from build123d import *

# Parameters (mm, degrees)
SKETCH_1_W          = 15
SKETCH_1_H          = 15
SKETCH_1_W_2        = 13
SKETCH_1_H_2        = 13
EXTRUDE_1_DEPTH     = 390
SKETCH_2_R          = 1.45
CUT_EXTRUDE_1_DEPTH = 391.36041039
SKETCH_3_R          = 1.45
CUT_EXTRUDE_2_DEPTH = 391.36041039


with BuildPart() as part:
    # 草图1 → 凸台-拉伸1 (new body)
    with BuildSketch(Plane(origin=(0, 0, 0), x_dir=(0, 0, -1), z_dir=(1, 0, 0))):
        Rectangle(SKETCH_1_W, SKETCH_1_H)
        Rectangle(SKETCH_1_W_2, SKETCH_1_H_2, mode=Mode.SUBTRACT)
    extrude(amount=EXTRUDE_1_DEPTH)

    # 草图2 → 切除-拉伸1 (cut, through all)
    with BuildSketch(Plane(origin=(0, 0, -7.5), x_dir=(-1, 0, 0), z_dir=(0, 0, -1))):
        with Locations((-366, 0)):
            Circle(SKETCH_2_R)
        with Locations((-376, 0)):
            Circle(SKETCH_2_R)
        with Locations((-19, 0)):
            Circle(SKETCH_2_R)
        with Locations((-9, 0)):
            Circle(SKETCH_2_R)
    extrude(amount=-CUT_EXTRUDE_1_DEPTH, mode=Mode.SUBTRACT)

    # 草图3 → 切除-拉伸2 (cut, through all)
    with BuildSketch(Plane(origin=(0, 7.5, 0), x_dir=(1, 0, 0), z_dir=(0, 1, 0))):
        with Locations(Location((371, 0, 0), (0, 0, 270))):
            Circle(SKETCH_3_R)
        with Locations(Location((381, 0, 0), (0, 0, 270))):
            Circle(SKETCH_3_R)
        with Locations(Location((14, 0, 0), (0, 0, 270))):
            Circle(SKETCH_3_R)
        with Locations(Location((177, 0, 0), (0, 0, 270))):
            Circle(SKETCH_3_R)
        with Locations(Location((187, 0, 0), (0, 0, 270))):
            Circle(SKETCH_3_R)
    extrude(amount=-CUT_EXTRUDE_2_DEPTH, mode=Mode.SUBTRACT)


solid = part.part
Here's how the part is built. I have some questions about the finished solid (model axes, mm). A direction names the side the tool comes from. Round coordinates to 2 decimals unless told otherwise and drop trailing zeros. Order: outer loops, then holes, each group sorted by start corner. A loop starts at its lowest first (then second) coordinate and runs counter-clockwise, first axis right, second up. Notation, with made-up numbers: M 20.25,-38.5 L 58.25,-38.5 A11 ccw 58.25,-27.5 Z; hole C 75,67.25 d7. An arc over 180 degrees is marked long. Return JSON: item names as keys, results as strings. Group by question number.
1. I'm going to push flat-ended pins straight in: pin 1 Ø3.5 at (x, z) = (381, 0) entering from -Y; pin 2 Ø2.5 at (x, y) = (19, 0) entering from -Z. Where does each tip first touch, or does it pass through?
2. If we section it at A-A on y = 4: List the corners of the cut face in (x, z) for me.
3. On a 3-axis mill with a long thin cutter (end or side, diameter ignored), from which of +Z, -Z, +X, -X, +Y, -Y can I reach the whole of each face in a straight line? I mean faces 5 (the face through (192, 0, 7.5)), 6 (the face through (192, 0, 6.5)). Say none if no direction works.
4. If we section it at B-B on x = 266: List the corners of the cut face in (y, z) for me, then the cut area to 3 significant figures.
5. Please list where these lines run through material, in increasing order: probe 1 along X at (y, z) = (6.8, 0); probe 2 along Y at (x, z) = (19.5, 0); probe 3 along Y at (x, z) = (9, 6.9).
6. If we mould it in two halves opening along Y, with no side actions, what happens to faces 1 (the face through (192, 6.5, 0)), 2 (the face through (192, -7.5, 0)), 3 (the face through (192, -6.5, 0)), 4 (the face through (0, 0, 7))? For each: pulls with the +Y half, pulls with the -Y half, needs draft (parallel to the pull), parting line crosses it, or undercut.
Reply:
{
 "1": {"pin 1": "y = -7.5", "pin 2": "through"},
 "2": {"outline": "M 0,-7.5 L 390,-7.5 L 390,-6.5 L 0,-6.5 Z; M 0,6.5 L 390,6.5 L 390,7.5 L 0,7.5 Z"},
 "3": {"face 5": "+Z, +X, -X, +Y, -Y", "face 6": "+X, -X"},
 "4": {"outline": "M -7.5,-7.5 L 7.5,-7.5 L 7.5,7.5 L -7.5,7.5 Z; hole M -6.5,-6.5 L 6.5,-6.5 L 6.5,6.5 L -6.5,6.5 Z", "area": "56.0 mm^2"},
 "5": {"probe 1": "0 to 12.55, 15.45 to 175.55, 178.45 to 185.55, 188.45 to 369.55, 372.45 to 379.55, 382.45 to 390", "probe 2": "-7.5 to -6.5, 6.5 to 7.5", "probe 3": "-7.5 to -1.45, 1.45 to 7.5"},
 "6": {"face 1": "undercut", "face 2": "pulls with the -Y half", "face 3": "undercut", "face 4": "needs draft"}
}
